Verification items for this drawing (mm, ordinates from the low corner). Give positions to 0.01 mm unless a question says otherwise; leave off trailing zeros. Write each loop counter-clockwise with the first axis right and the second up, starting at its lowest first coordinate (ties: lowest second). Pieces come first, ordered by that corner, then holes. Notation, with made-up numbers: (19.5, 22) -> (61.5, 22) arc R22 ccw to (61.5, 32) -> close; hole circle Ø2 at (-39.75, 16). An arc over 180 degrees is marked (long way). One line per item, written item: value.
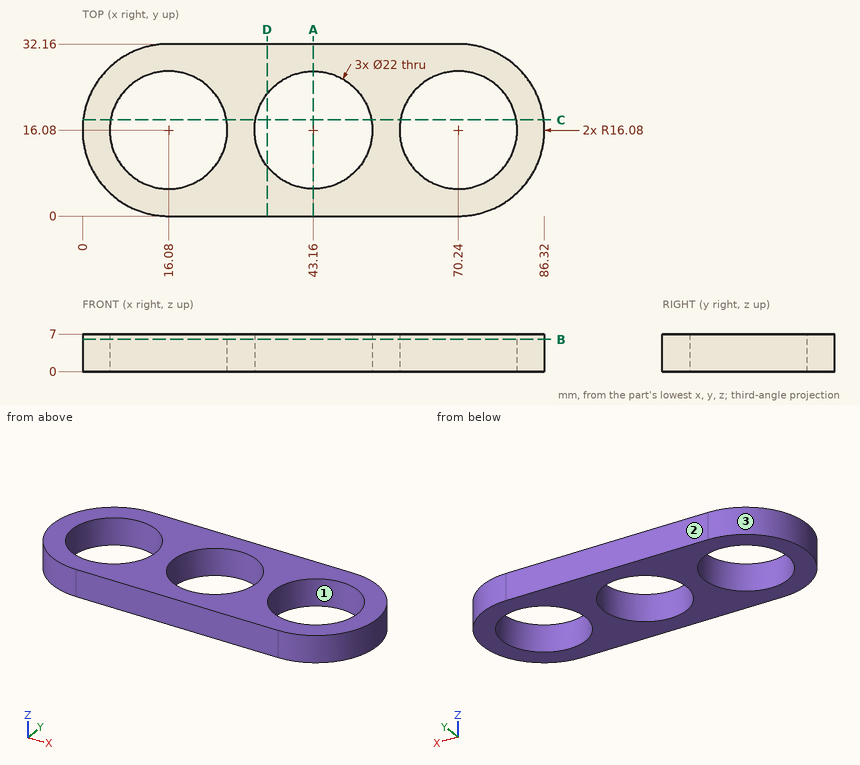
1) Sectioned sample at C-C on y = 18. Record the cut outline in (x, z), plus the area to 3 significant figures.
Verdict:
outline: (0.12, 0) -> (5.25, 0) -> (5.25, 7) -> (0.12, 7) -> close; (26.91, 0) -> (32.33, 0) -> (32.33, 7) -> (26.91, 7) -> close; (53.99, 0) -> (59.41, 0) -> (59.41, 7) -> (53.99, 7) -> close; (81.07, 0) -> (86.2, 0) -> (86.2, 7) -> (81.07, 7) -> close
area: 148 mm^2
2) Scan lines: probe 1 along Y at (x, z) = (70.24, 4.75); probe 2 along X at (y, z) = (21, 2); probe 3 along X at (y, z) = (23, 2). Record each from-to range of solid material in increasing order.
Verdict:
probe 1: 0 to 5.08, 27.08 to 32.16
probe 2: 0.77 to 6.24, 25.92 to 33.32, 53 to 60.4, 80.08 to 85.55
probe 3: 1.57 to 7.53, 24.63 to 34.61, 51.71 to 61.69, 78.79 to 84.75
3) Mould release check, pull along X, two halves, no side actions. Record for the marked faces 1, 2 and 3: released by +X, released by -X, zero draft, split by the parting line, or undercut.
Verdict:
face 1: undercut
face 2: zero draft
face 3: released by -X
4) Sectioned sample at B-B on z = 6. Record the cut outline in (x, y).
Verdict:
outline: (16.08, 0) -> (70.24, 0) arc R16.08 ccw to (70.24, 32.16) -> (16.08, 32.16) arc R16.08 ccw to start; hole circle Ø22 at (16.08, 16.08); hole circle Ø22 at (43.16, 16.08); hole circle Ø22 at (70.24, 16.08)
5) Sectioned sample at D-D on x = 34.5. Record the cut outline in (y, z), plus the area to 3 significant figures.
Verdict:
outline: (0, 0) -> (9.3, 0) -> (9.3, 7) -> (0, 7) -> close; (22.86, 0) -> (32.16, 0) -> (32.16, 7) -> (22.86, 7) -> close
area: 130 mm^2
6) Sectioned sample at A-A on x = 43.16. Record the cut outline in (y, z), plus the area to 3 significant figures.
Verdict:
outline: (0, 0) -> (5.08, 0) -> (5.08, 7) -> (0, 7) -> close; (27.08, 0) -> (32.16, 0) -> (32.16, 7) -> (27.08, 7) -> close
area: 71.1 mm^2
